Geometry check sheet. Reference: the model listing, model coordinates, mm. Face numbers are marked on the shaded views. Round coordinates to 2 decimals unless told otherwise and drop trailing zeros. Order: outer loops, then holes, each group sorted by start corner. A loop starts at its lowest first (then second) coordinate and runs counter-clockwise, first axis right, second up. Notation, with made-up numbers: (59.5, 82) -> (73.5, 82) arc R27 cw to (73.5, 104) -> close; hole circle Ø2 at (-40, 45). An arc over 180 degrees is marked (long way). Answer as a JSON object with one key per item and string values. Group by question number.
from build123d import *

# Parameters (mm, degrees)
F_4_40_TAPPED_HOLE1_REACH  = 199.542
F_4_40_TAPPED_HOLE1_BORE_R = 1.1303
CIRPATTERN1_COUNT          = 3


# Read off the part's stored shape, not the designer's step: CSK for #4 Flat Head Machine Screw (100)1
with BuildPart() as part:
    # Sketch1 → Revolve1 (revolve)
    with BuildSketch(Plane.XY, mode=Mode.PRIVATE) as revolve1_sk:
        Polygon((-76.2, 0), (-81.8896, 0), (-81.8896, -7.6708), (-83.82, -7.6708), (-83.82, -71.1708), (-76.2, -71.1708), align=None)
    revolve(revolve1_sk.sketch.rotate(Axis((0, 0, 0), (0, 1, 0)), 270), axis=Axis((0, 0, 0), (0, 1, 0)))

    # #4-40 Tapped Hole1 bore (on position points) → #4-40 Tapped Hole1 (cut, up to next)
    with BuildSketch(Plane(origin=(81.8896, -3.81, 0), x_dir=(0, 0, 1), z_dir=(1, 0, 0)), mode=Mode.PRIVATE) as f_4_40_tapped_hole1_sk1:
        Circle(F_4_40_TAPPED_HOLE1_BORE_R)
    f_4_40_tapped_hole1_tool1 = extrude(f_4_40_tapped_hole1_sk1.sketch, amount=-F_4_40_TAPPED_HOLE1_REACH, mode=Mode.PRIVATE) & part.part
    f_4_40_tapped_hole1 = f_4_40_tapped_hole1_tool1.solids().sort_by_distance((81.8896, -3.81, 0))[0]
    add(f_4_40_tapped_hole1, mode=Mode.SUBTRACT)

    # CSK for _4 Flat Head Machine Screw _ 2 → CSK for #4 Flat Head Machine Screw (100)1 (revolve, cut)
    with BuildSketch(Plane(origin=(0, -67.3608, 0), x_dir=(0, 1, 0), z_dir=(0, 0, -1))):
        Polygon((2.857519918, 83.820016713), (0, 83.820016713), (0, 76.182513139), (1.63195, 76.182513139), (1.63195, 82.791641447), align=None)
    csk_for_4_flat_head_machine_screw_100 = revolve(axis=Axis((0, -67.3608, 0), (1, 0, 0)), mode=Mode.SUBTRACT)

    # CirPattern1: #4-40 Tapped Hole1, CSK for #4 Flat Head Machine Screw (100)1 ×3 about axis
    cirpattern1_axis = Axis((0, 0, 0), (0, -1, 0))
    add([f_4_40_tapped_hole1.rotate(cirpattern1_axis, i * 360 / CIRPATTERN1_COUNT) for i in range(1, CIRPATTERN1_COUNT)], mode=Mode.SUBTRACT)
    add([csk_for_4_flat_head_machine_screw_100.rotate(cirpattern1_axis, i * 360 / CIRPATTERN1_COUNT) for i in range(1, CIRPATTERN1_COUNT)], mode=Mode.SUBTRACT)


solid = part.part
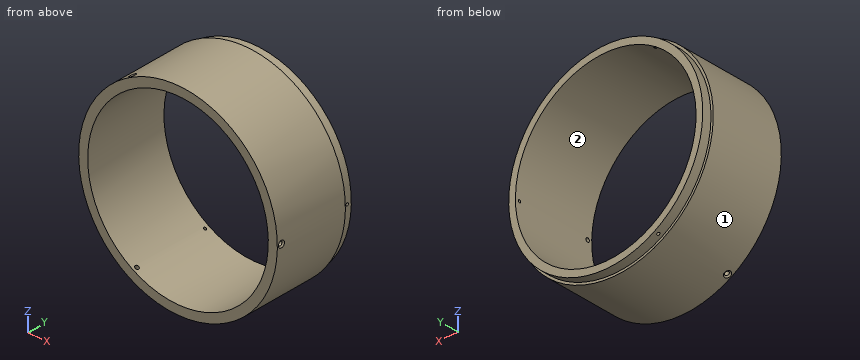
Item 1: Sectioned sample at B-B, the plane z = 47. Enter the section's corners in (x, y), then the cut area to 3 significant figures.
Item 2: Depth check by flat-ended pin: pin 1 Ø2 at (y, z) = (-29.5, -18) entering from -X; pin 2 Ø5 at (y, z) = (-47.5, -30.5) entering from +X (3 decimals); pin 3 Ø5 at (y, z) = (-48.5, -37) entering from +X. Enter the tip coordinate at first touch or a pass-through.
Item 3: Mould release check, pull along X, two halves, no side actions. Record for the marked faces 1 and 2: pulls with the +X half, pulls with the -X half, needs draft (parallel to the pull), parting line crosses it, or undercut.
Item 4: Sectioned sample at C-C, the plane y = -26. Enter the section's corners in (x, z).
Item 5: Thickness scan on L1, parallel to Y at x = 78.25, z = 0; L2, parallel to Z at x = -1.5, y = -17.5; L3, parallel to X at y = -20.5, z = 0. Record the ranges inside material, lowest first.
Item 6: Sectioned sample at A-A, the plane x = 0. Enter the section's corners in (y, z), then the cut area to 3 significant figures.
Result:
{
 "1": {"outline": "(-69.4, -71.17) -> (-59.98, -71.17) -> (-59.98, 0) -> (-67.06, 0) -> (-67.06, -7.67) -> (-69.4, -7.67) -> close; (59.98, -71.17) -> (69.4, -71.17) -> (69.4, -7.67) -> (67.06, -7.67) -> (67.06, 0) -> (59.98, 0) -> close", "area": "1,310 mm2"},
 "2": {"pin 1": "stops at x = -82.08", "pin 2": "stops at x = 79.005", "pin 3": "stops at x = 76.39"},
 "3": {"face 1": "parting line crosses it", "face 2": "undercut"},
 "4": {"outline": "circle Ø167.64 at (0, 0); hole circle Ø152.4 at (0, 0)"},
 "5": {"L1": "y = -71.17 to -68.99, -65.73 to -4.94, -2.68 to 0", "L2": "z = -83.81 to -76.19, 76.19 to 83.81", "L3": "x = -83.82 to -76.2, 76.2 to 83.82"},
 "6": {"outline": "(-71.17, -83.82) -> (-7.67, -83.82) -> (-7.67, -81.89) -> (0, -81.89) -> (0, -76.2) -> (-71.17, -76.2) -> close; (-71.17, 76.2) -> (0, 76.2) -> (0, 81.89) -> (-7.67, 81.89) -> (-7.67, 83.82) -> (-71.17, 83.82) -> close", "area": "1,060 mm2"}
}
